Autodesk Inventor part; units mm, degrees
ref_plane "YZ Plane" through (0, 0, 0) normal (1, 0, 0) x (0, 1, 0)
ref_plane "XZ Plane" through (0, 0, 0) normal (0, 1, 0) x (-1, 0, 0)
ref_plane "XY Plane" through (0, 0, 0) normal (0, 0, 1) x (1, 0, 0)
sketch "Esquisse1" plane through (0, 0, 0) normal (1, 0, 0) x (0, 1, 0)
  line L0 (0.5, 12) -> (-0.5, 12)
  line L1 (-0.5, 12) -> (-0.5, -12)
  line L2 (-0.5, -12) -> (0.5, -12)
  line L3 (0.5, -12) -> (0.5, 12)
  line L4 (0.5, 12) -> (-0.5, -12) construction
  line L5 (-0.5, 12) -> (0.5, -12) construction
  line L6 (0.5, -12) -> (-4.7, -12)
  line L7 (-4.7, -12) -> (-4.7, -13)
  line L8 (-4.7, -13) -> (0.5, -13)
  line L9 (0.5, -13) -> (0.5, -12)
  line L10 (0.5, 12) -> (-4.7, 12)
  line L11 (-4.7, 12) -> (-4.7, 13)
  line L12 (-4.7, 13) -> (0.5, 13)
  line L13 (0.5, 13) -> (0.5, 12)
  line L14 (-4.7, -13) -> (-3.7, -13)
  line L15 (-3.7, -13) -> (-3.7, -21)
  line L16 (-3.7, -21) -> (-4.7, -21)
  line L17 (-4.7, -21) -> (-4.7, -13)
  line L18 (-4.7, 13) -> (-3.7, 13)
  line L19 (-3.7, 13) -> (-3.7, 21)
  line L20 (-3.7, 21) -> (-4.7, 21)
  line L21 (-4.7, 21) -> (-4.7, 13)
  point P0 (0, 0)
  dimension "d0" = 24
  dimension "d1" = 1
  dimension "d2" = 8
  dimension "d3" = 4.2
extrude "Extrusion1" add sketch "Esquisse1" along normal mid plane 15.8
sketch "Esquisse2" plane through (-7.9, -0.5, -12) normal (0, -1, 0) x (1, 0, 0)
  circle A0 centre (7.9, 19.9) radius 2.1
  line L0 (7.9, 19.9) -> (7.9, 12) construction
  line L1 (7.9, 12) -> (7.9, 4.1) construction
  line L2 (10, 19.9) -> (10, 24)
  line L3 (0, 24) -> (15.8, 24)
  line L4 (5.8, 24) -> (5.8, 19.9)
  line L5 (10, 19.9) -> (5.8, 19.9) construction
  dimension "d6" = 15.8
  dimension "d7" = 4.2
extrude "Extrusion2" cut sketch "Esquisse2" against normal through all
sketch "Esquisse3" plane through (-7.9, -3.7, 21) normal (0, 1, 0) x (1, 0, 0)
  circle A0 centre (7.9, 4) radius 1.6
  line L0 (0, 0) -> (15.8, 0) construction
  line L1 (7.9, 0) -> (7.9, 4) construction
  line L2 (7.9, 4) -> (7.9, 8) construction
  line L3 (0, 8) -> (15.8, 8) construction
  point P0 (7.9, 21)
  dimension "d10" = 3.2
extrude "Extrusion3" cut sketch "Esquisse3" against normal through all
mirror "Symétrie2" about plane through (0, 0, 0) normal (0, 0, 1) of "Extrusion2", "Extrusion3"
sketch "Sketch4" plane through (7.9, 0, 0) normal (1, 0, 0) x (0, 0, -1)
  line L0 (13, 0.5) -> (-13, 0.5)
  line L1 (-13, 0.5) -> (-13, -3.7)
  line L2 (-13, -3.7) -> (-21, -3.7)
  line L3 (-21, -3.7) -> (-21, -4.7)
  line L4 (-21, -4.7) -> (-12, -4.7)
  line L5 (-12, -4.7) -> (-12, -0.5)
  line L6 (-12, -0.5) -> (12, -0.5)
  line L7 (12, -0.5) -> (12, -4.7)
  line L8 (12, -4.7) -> (21, -4.7)
  line L9 (21, -4.7) -> (21, -3.7)
  line L10 (21, -3.7) -> (13, -3.7)
  line L11 (13, -3.7) -> (13, 0.5)
  line L12 (-12, -0.5) -> (-13, -0.5)
  line L13 (12, -0.5) -> (13, -0.5)
  point P0 (0, 0)
extrude "Extrusion4" cut sketch "Sketch4" against normal through all contours L11 L10 L9 L8 L7 L13 | L12 L5 L4 L3 L2 L1
sketch "Sketch5" plane through (-7.9, 0.5, 13) normal (0, 1, 0) x (1, 0, 0)
  line L0 (-4.1, 0) -> (19.9, 0)
  line L1 (19.9, 0) -> (19.9, 26)
  line L2 (19.9, 26) -> (-4.1, 26)
  line L3 (-4.1, 26) -> (-4.1, 0)
  line L4 (-4.1, 0) -> (19.9, 26) construction
  line L5 (19.9, 0) -> (-4.1, 26) construction
  arc A0 (5.8, 20.9) -> (10, 20.9) centre (7.9, 20.9) ccw
  line L6 (5.8, 20.9) -> (5.8, 25)
  line L7 (5.8, 25) -> (10, 25)
  line L8 (10, 25) -> (10, 20.9)
  line L9 (10, 1) -> (5.8, 1)
  line L10 (5.8, 1) -> (5.8, 5.1)
  arc A1 (10, 5.1) -> (5.8, 5.1) centre (7.9, 5.1) ccw
  line L11 (10, 5.1) -> (10, 1)
  line L12 (0, 0) -> (15.8, 0)
  line L13 (15.8, 26) -> (15.8, 0)
  line L14 (15.8, 26) -> (0, 26)
  line L15 (0, 0) -> (0, 26)
  point P0 (7.9, 13)
  dimension "d16" = 24
  dimension "d22" = 26
extrude "Extrusion5" add sketch "Sketch5" against normal up to surface (1 mm away) contours L3 L2 L15 L0 | L13 L2 L1 L0
sketch "Sketch7" plane through (-12, 0.5, -13) normal (0, 1, 0) x (1, 0, 0)
  circle A0 centre (12, -13) radius 9
  dimension "d23" = 18
extrude "Extrusion7" cut sketch "Sketch7" against normal through all
sketch "Sketch8" plane through (12, 0.5, 13) normal (0, 1, 0) x (1, 0, 0)
  line L0 (-24, 0) -> (0, 0)
  line L1 (0, 0) -> (0, 26)
  line L2 (0, 26) -> (-24, 26)
  line L3 (-24, 26) -> (-24, 0)
  arc A0 (-9.9, 4.2484) -> (-9.9, 21.7516) centre (-12, 13) ccw
  line L4 (-9.9, 4.2484) -> (-9.9, 1)
  line L5 (-9.9, 1) -> (-14.1, 1)
  line L6 (-14.1, 1) -> (-14.1, 4.2484)
  arc A1 (-14.1, 21.7516) -> (-14.1, 4.2484) centre (-12, 13) ccw
  line L7 (-14.1, 21.7516) -> (-14.1, 25)
  line L8 (-14.1, 25) -> (-9.9, 25)
  line L9 (-9.9, 25) -> (-9.9, 21.7516)
  line L10 (-14.1, 2) -> (-9.9, 2)
  line L11 (-14.1, 24) -> (-9.9, 24)
  line L12 (-12, 2) -> (-12, 1) construction
  line L13 (-12, 24) -> (-12, 25) construction
  point P0 (-14.1, 24)
  dimension "d27" = 1
extrude "Extrusion9" add sketch "Sketch8" against normal up to surface (1 mm away) contours L4 L5 L6 L10 | L11 L7 L8 L9
sketch "Sketch9" plane through (12, 0.5, 13) normal (0, 1, 0) x (1, 0, 0)
  line L0 (-24, 0) -> (0, 0)
  line L1 (0, 0) -> (0, 26)
  line L2 (0, 26) -> (-24, 26)
  line L3 (-24, 26) -> (-24, 0)
  arc A0 (-9.9, 4.2484) -> (-9.9, 21.7516) centre (-12, 13) ccw
  line L4 (-9.9, 4.2484) -> (-9.9, 2)
  line L5 (-9.9, 2) -> (-14.1, 2)
  line L6 (-14.1, 2) -> (-14.1, 4.2484)
  arc A1 (-14.1, 21.7516) -> (-14.1, 4.2484) centre (-12, 13) ccw
  line L7 (-14.1, 21.7516) -> (-14.1, 24)
  line L8 (-14.1, 24) -> (-9.9, 24)
  line L9 (-9.9, 24) -> (-9.9, 21.7516)
  line L10 (0, 26) -> (-4.1, 26)
  line L11 (-4.1, 26) -> (-4.1, 0)
  line L12 (-4.1, 0) -> (0, 0)
  line L13 (0, 0) -> (0, 26)
  point P0 (-4.1, 8.6884)
  point P1 (-4.1, 17.3116)
  dimension "d32" = 4.1
extrude "Extrusion10" cut sketch "Sketch9" against normal through all contours L11 A0 L2 L1 L0
fillet "Fillet3" radius 1 2 edges at (7.9, 0, 4.3116) (7.9, 0, -4.3116)
properties part number "Adapt_Roue_libre"
Here's how the part is built. I have some questions about the finished solid (model axes, mm). A direction names the side the tool comes from. Give positions to 0.01 mm unless a question says otherwise; leave off trailing zeros. Loops run counter-clockwise (first coordinate to the right, second up) from the corner with the lowest first, then second, coordinate; pieces in that order, holes last. Notation, with made-up numbers: (87, -24.5) -> (141, -24.5) arc R27 ccw to (141, -2.5) -> close; hole circle Ø9 at (-10.75, 75). An arc over 180 degrees is marked (long way). Use one line per item in the form item = value. Start each with the question number.
1) Imagine slicing it at C-C (y = 0.35). Please give me the cut outline in (x, z).
2) Thinking about a two-plate mould opening in Z: for faces 1 (the face through (7.9, 0, 10)), 2 (the face through (-2, 0, 13)), 3 (the face through (2.1, 0, 10)), 4 (the face through (0, 0, 11)), which applies, +Z half, -Z half, draft (parallel to the pull), parting line (faces both ways), or undercut?
3) Imagine slicing it at B-B (z = -9.25). Please give me the cut outline in (x, y), then the cut area to 3 significant figures.
4) Please list where these lines run through material, in increasing order: line 1 along X through (y, z) = (0.4, -9); line 2 along Z through (x, y) = (1.75, 0.4); line 3 along Z through (x, y) = (7.25, -0.4).
5) Imagine slicing it at A-A (x = -1). Please give me the cut outline in (y, z).
6) Which directions (+Z, -Z, +X, -X, +Y, -Y) give clear straight access to the entire face, cutting with the end or side of a thin tool? Please do faces 5 (the face through (0, 0, -11)), 6 (the face through (-2, 0, -13)).
7) Imagine slicing it at D-D (z = -1). Please give me the cut outline in (x, y), then the cut area to 3 significant figures.
Check values:
q1.outline = (-12, -13) -> (7.9, -13) -> (7.9, -7.24) arc R1 ccw to (6.21, -6.51) arc R9 cw to (2.1, -8.75) -> (2.1, -11) -> (-2.1, -11) -> (-2.1, -8.75) arc R9 cw to (-2.1, 8.75) -> (-2.1, 11) -> (2.1, 11) -> (2.1, 8.75) arc R9 cw to (6.21, 6.51) arc R1 ccw to (7.9, 7.24) -> (7.9, 13) -> (-12, 13) -> close
q2.face_1 = draft
q2.face_2 = +Z half
q2.face_3 = undercut
q2.face_4 = undercut
q3.outline = (-12, -0.5) -> (-2.1, -0.5) -> (-2.1, 0.5) -> (-12, 0.5) -> close; (2.1, -0.5) -> (7.9, -0.5) -> (7.9, 0.5) -> (2.1, 0.5) -> close
q3.area = 15.7 mm^2
q4.line_1 = -12 to -2.1, 2.1 to 7.9
q4.line_2 = -13 to -11, 11 to 13
q4.line_3 = -13 to -6.3, 6.3 to 13
q5.outline = (-0.5, -13) -> (0.5, -13) -> (0.5, -11) -> (-0.5, -11) -> close; (-0.5, 11) -> (0.5, 11) -> (0.5, 13) -> (-0.5, 13) -> close
q6.face_5 = +Y, -Y
q6.face_6 = -Z, +X, -X, +Y, -Y
q7.outline = (-12, -0.5) -> (-8.94, -0.5) -> (-8.94, 0.5) -> (-12, 0.5) -> close
q7.area = 3.06 mm^2
